from build123d import *

# Parameters (mm, degrees)
SKETCH3_W           = 150
SKETCH3_H           = 150
SKETCH3_R           = 1.75
SKETCH3_R_2         = 1.5
BOSS_EXTRUDE2_DEPTH = 3
CUT_EXTRUDE2_REACH  = 5
FILLET2_R           = 5
FILLET3_R           = 20


with BuildPart() as part:
    # Sketch3 → Boss-Extrude2 (new body)
    with BuildSketch(Plane(origin=(0, 0, 0), x_dir=(1, 0, 0), z_dir=(0, 1, 0))):
        Rectangle(SKETCH3_W, SKETCH3_H)
        with Locations((-70, 70)):
            Circle(SKETCH3_R, mode=Mode.SUBTRACT)
        with Locations((70, -70)):
            Circle(SKETCH3_R, mode=Mode.SUBTRACT)
        with Locations((-70, -70)):
            Circle(SKETCH3_R, mode=Mode.SUBTRACT)
        with Locations((70, 70)):
            Circle(SKETCH3_R, mode=Mode.SUBTRACT)
        with Locations((-10, 10)):
            Circle(SKETCH3_R_2, mode=Mode.SUBTRACT)
        with Locations((10, -10)):
            Circle(SKETCH3_R_2, mode=Mode.SUBTRACT)
        with Locations((-10, -10)):
            Circle(SKETCH3_R_2, mode=Mode.SUBTRACT)
        with Locations((10, 10)):
            Circle(SKETCH3_R_2, mode=Mode.SUBTRACT)
    extrude(amount=BOSS_EXTRUDE2_DEPTH)

    # Sketch4 → Cut-Extrude2 (cut, up to next)
    with BuildSketch(Plane(origin=(0, 3, 0), x_dir=(1, 0, 0), z_dir=(0, 1, 0)), mode=Mode.PRIVATE) as cut_extrude2_sk1:
        with BuildLine():
            Line((-27.67766953, 20.606601718), (-65.050252532, 57.97918472))
            ThreePointArc((-65.050252532, 57.97918472), (-65.050252532, 65.050252532), (-57.97918472, 65.050252532))
            Line((-57.97918472, 65.050252532), (-20.606601718, 27.67766953))
            ThreePointArc((-20.606601718, 27.67766953), (-20.606601718, 20.606601718), (-27.67766953, 20.606601718))
        make_face()
    cut_extrude2_tool1 = extrude(cut_extrude2_sk1.sketch, amount=-CUT_EXTRUDE2_REACH, mode=Mode.PRIVATE) & part.part
    add(cut_extrude2_tool1.solids().sort_by_distance((-42.828427, 3, -42.828427))[0], mode=Mode.SUBTRACT)
    # Sketch4 → Cut-Extrude2 (cut, up to next)
    with BuildSketch(Plane(origin=(0, 3, 0), x_dir=(1, 0, 0), z_dir=(0, 1, 0)), mode=Mode.PRIVATE) as cut_extrude2_sk2:
        Polygon((-75, 60.857864376), (-14.142135624, 0), (-75, -60.857864376), align=None)
    cut_extrude2_tool2 = extrude(cut_extrude2_sk2.sketch, amount=-CUT_EXTRUDE2_REACH, mode=Mode.PRIVATE) & part.part
    add(cut_extrude2_tool2.solids().sort_by_distance((-54.714045, 3, 0))[0], mode=Mode.SUBTRACT)
    # Sketch4 → Cut-Extrude2 (cut, up to next)
    with BuildSketch(Plane(origin=(0, 3, 0), x_dir=(1, 0, 0), z_dir=(0, 1, 0)), mode=Mode.PRIVATE) as cut_extrude2_sk3:
        with BuildLine():
            Line((27.67766953, 20.606601718), (65.050252532, 57.97918472))
            ThreePointArc((65.050252532, 57.97918472), (65.050252532, 65.050252532), (57.97918472, 65.050252532))
            Line((57.97918472, 65.050252532), (20.606601718, 27.67766953))
            ThreePointArc((20.606601718, 27.67766953), (20.606601718, 20.606601718), (27.67766953, 20.606601718))
        make_face()
    cut_extrude2_tool3 = extrude(cut_extrude2_sk3.sketch, amount=-CUT_EXTRUDE2_REACH, mode=Mode.PRIVATE) & part.part
    add(cut_extrude2_tool3.solids().sort_by_distance((42.828427, 3, -42.828427))[0], mode=Mode.SUBTRACT)
    # Sketch4 → Cut-Extrude2 (cut, up to next)
    with BuildSketch(Plane(origin=(0, 3, 0), x_dir=(1, 0, 0), z_dir=(0, 1, 0)), mode=Mode.PRIVATE) as cut_extrude2_sk4:
        with BuildLine():
            Line((27.67766953, -20.606601718), (65.050252532, -57.97918472))
            ThreePointArc((65.050252532, -57.97918472), (65.050252532, -65.050252532), (57.97918472, -65.050252532))
            Line((57.97918472, -65.050252532), (20.606601718, -27.67766953))
            ThreePointArc((20.606601718, -27.67766953), (20.606601718, -20.606601718), (27.67766953, -20.606601718))
        make_face()
    cut_extrude2_tool4 = extrude(cut_extrude2_sk4.sketch, amount=-CUT_EXTRUDE2_REACH, mode=Mode.PRIVATE) & part.part
    add(cut_extrude2_tool4.solids().sort_by_distance((42.828427, 3, 42.828427))[0], mode=Mode.SUBTRACT)
    # Sketch4 → Cut-Extrude2 (cut, up to next)
    with BuildSketch(Plane(origin=(0, 3, 0), x_dir=(1, 0, 0), z_dir=(0, 1, 0)), mode=Mode.PRIVATE) as cut_extrude2_sk5:
        with BuildLine():
            Line((-27.67766953, -20.606601718), (-65.050252532, -57.97918472))
            ThreePointArc((-65.050252532, -57.97918472), (-65.050252532, -65.050252532), (-57.97918472, -65.050252532))
            Line((-57.97918472, -65.050252532), (-20.606601718, -27.67766953))
            ThreePointArc((-20.606601718, -27.67766953), (-20.606601718, -20.606601718), (-27.67766953, -20.606601718))
        make_face()
    cut_extrude2_tool5 = extrude(cut_extrude2_sk5.sketch, amount=-CUT_EXTRUDE2_REACH, mode=Mode.PRIVATE) & part.part
    add(cut_extrude2_tool5.solids().sort_by_distance((-42.828427, 3, 42.828427))[0], mode=Mode.SUBTRACT)
    # Sketch4 → Cut-Extrude2 (cut, up to next)
    with BuildSketch(Plane(origin=(0, 3, 0), x_dir=(1, 0, 0), z_dir=(0, 1, 0)), mode=Mode.PRIVATE) as cut_extrude2_sk6:
        Polygon((75, 60.857864376), (14.142135624, 0), (75, -60.857864376), align=None)
    cut_extrude2_tool6 = extrude(cut_extrude2_sk6.sketch, amount=-CUT_EXTRUDE2_REACH, mode=Mode.PRIVATE) & part.part
    add(cut_extrude2_tool6.solids().sort_by_distance((54.714045, 3, 0))[0], mode=Mode.SUBTRACT)
    # Sketch4 → Cut-Extrude2 (cut, up to next)
    with BuildSketch(Plane(origin=(0, 3, 0), x_dir=(1, 0, 0), z_dir=(0, 1, 0)), mode=Mode.PRIVATE) as cut_extrude2_sk7:
        Polygon((-60.857864376, -75), (60.857864376, -75), (0, -14.142135624), align=None)
    cut_extrude2_tool7 = extrude(cut_extrude2_sk7.sketch, amount=-CUT_EXTRUDE2_REACH, mode=Mode.PRIVATE) & part.part
    add(cut_extrude2_tool7.solids().sort_by_distance((0, 3, 54.714045))[0], mode=Mode.SUBTRACT)
    # Sketch4 → Cut-Extrude2 (cut, up to next)
    with BuildSketch(Plane(origin=(0, 3, 0), x_dir=(1, 0, 0), z_dir=(0, 1, 0)), mode=Mode.PRIVATE) as cut_extrude2_sk8:
        Polygon((-60.857864376, 75), (0, 14.142135624), (60.857864376, 75), align=None)
    cut_extrude2_tool8 = extrude(cut_extrude2_sk8.sketch, amount=-CUT_EXTRUDE2_REACH, mode=Mode.PRIVATE) & part.part
    add(cut_extrude2_tool8.solids().sort_by_distance((0, 3, -54.714045))[0], mode=Mode.SUBTRACT)

    # Fillet2
    fillet2_edges = [part.edges().sort_by_distance(p)[0] for p in [
        (75, 1.5, 75),
        (-75, 1.5, 75),
        (-75, 1.5, -75),
        (75, 1.5, -75),
    ]]
    fillet(fillet2_edges, radius=FILLET2_R)

    # Fillet3
    fillet3_edges = [part.edges().sort_by_distance(p)[0] for p in [
        (75, 1.5, -60.857864376),
        (75, 1.5, 60.857864376),
        (14.142135624, 1.5, 0),
        (-60.857864376, 1.5, 75),
        (0, 1.5, 14.142135624),
        (60.857864376, 1.5, 75),
        (-75, 1.5, 60.857864376),
        (-75, 1.5, -60.857864376),
        (-14.142135624, 1.5, 0),
        (-60.857864376, 1.5, -75),
        (60.857864376, 1.5, -75),
        (0, 1.5, -14.142135624),
    ]]
    fillet(fillet3_edges, radius=FILLET3_R)


solid = part.part
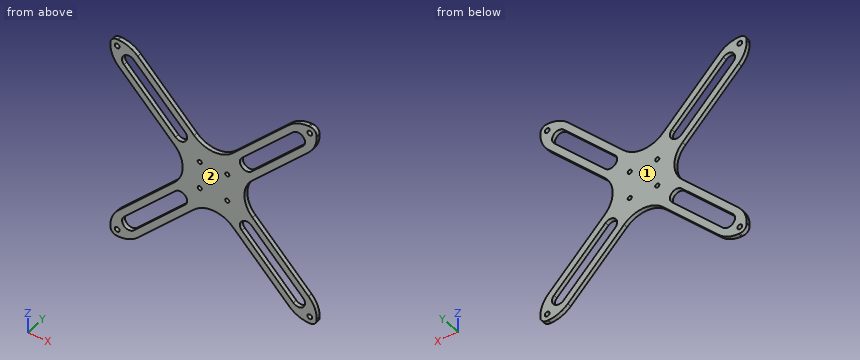
The model under review builds one solid part; all positions refer to its coordinate system, in mm. Face numbers are marked on the shaded views. Give positions to 0.01 mm unless a question says otherwise; leave off trailing zeros. Loops run counter-clockwise (first coordinate to the right, second up) from the corner with the lowest first, then second, coordinate; pieces in that order, holes last. Notation, with made-up numbers: (-26.75, 54.25) -> (20.25, 54.25) arc R26 cw to (20.25, 83.25) -> close; hole circle Ø4 at (-40, -8). An arc over 180 degrees is marked (long way). Write each question's results on one line, items separated by ' | '.
1) Take a section at A-A, the plane z = 34.5. Give the boundary of the cut face in (x, y), plus the area to 3 significant figures.
Conclusion:
outline: (-48.64, 0) -> (-41.57, 0) -> (-41.57, 3) -> (-48.64, 3) -> close; (-27.43, 0) -> (-20.36, 0) -> (-20.36, 3) -> (-27.43, 3) -> close; (20.36, 0) -> (27.43, 0) -> (27.43, 3) -> (20.36, 3) -> close; (41.57, 0) -> (48.64, 0) -> (48.64, 3) -> (41.57, 3) -> close | area: 84.9 mm^2
2) Take a section at D-D, the plane z = -3.5. Give the boundary of the cut face in (x, y).
Conclusion:
outline: (-22.74, 0) -> (22.74, 0) -> (22.74, 3) -> (-22.74, 3) -> close
3) Draft analysis for pull direction Y (two halves, no side actions). For the marked faces 1 and 2, state which applies: pulls with the +Y half, pulls with the -Y half, needs draft (parallel to the pull), parting line crosses it, or undercut.
Conclusion:
face 1: pulls with the +Y half | face 2: pulls with the -Y half
4) Take a section at B-B, the plane x = 49. Give the boundary of the cut face in (y, z), plus the area to 3 significant figures.
Conclusion:
outline: (0, -63.14) -> (3, -63.14) -> (3, -56.07) -> (0, -56.07) -> close; (0, -41.93) -> (3, -41.93) -> (3, -34.86) -> (0, -34.86) -> close; (0, 34.86) -> (3, 34.86) -> (3, 41.93) -> (0, 41.93) -> close; (0, 56.07) -> (3, 56.07) -> (3, 63.14) -> (0, 63.14) -> close | area: 84.9 mm^2
5) Insertion check: pin 1 Ø1.5 at (x, y) = (28, 2) entering from -Z; pin 2 Ø10 at (x, z) = (-25.5, 7) entering from +Y. Each pin has a flat end and moves straight along its axis. Give the tip position at first contact, or say it passes through.
Conclusion:
pin 1: stops at z = -42.89 | pin 2: stops at y = 3
6) For line 1 along X through (y, z) = (2, 70); line 2 along X through (y, z) = (0.95, -52.5); line 3 along Z through (x, y) = (-64, 2.85), list the stretches that pass through material, from the lowest coordinate up. Write a range as from..to.
Conclusion:
line 1: x = -75..-71.75, -68.25..-55.91, 55.91..68.25, 71.75..75 | line 2: x = -66.64..-59.57, -45.43..-38.36, 38.36..45.43, 59.57..66.64 | line 3: z = -74.33..-65.85, -56.93..-49.86, 49.86..56.93, 65.85..74.33
7) Take a section at C-C, the plane y = 2.3. Count the separate pieces of the cut face and the enclosed holes in it, plus the area to 3 significant figures.
Conclusion:
separate pieces: 1 | enclosed holes: 12 | area: 5,440 mm^2
